The model under review builds one solid part; all positions refer to its coordinate system, in mm. A direction names the side the tool comes from. Give positions to 0.01 mm unless a question says otherwise; leave off trailing zeros. Return JSON: item names as keys, results as strings. Group by question number.
from build123d import *

# Parameters (mm, degrees)
F0_R            = 5
F1_DEPTH        = 6.5
F2_R            = 2.9
F3_DEPTH        = 10
F4_W            = 1.5
F4_H            = 25.2303039929
F5_COPIES_COUNT = 8
F6_R            = 30.1842300119
F6_R_2          = 28.1532988992
F7_DEPTH        = 4.5
F8_R            = 1.5
F9_R            = 2.5
F10_DEPTH       = 3


# Not quite as in the source:
# - a pattern or mirror of a feature is missing from the dataset's text; its kind, count and spacing are read off the source's solid


with BuildPart() as f1:
    # F0 (on Top) → F1 (new body, symmetric)
    with BuildSketch(Plane.XY):
        Circle(F0_R)
    extrude(amount=F1_DEPTH, both=True)

    # F2 (on face) → F3 (cut)
    with BuildSketch(Plane(origin=(0, 0, -6.5), x_dir=(1, 0, 0), z_dir=(0, 0, -1))):
        Circle(F2_R)
    extrude(amount=-F3_DEPTH, mode=Mode.SUBTRACT)

    # F4 (on Top) → F5 (revolve)
    with BuildSketch(Plane.XY):
        with Locations((-0.75, -17.3848480035)):
            Rectangle(F4_W, F4_H)
    f5 = revolve(axis=Axis((0, -23.260904476, 0), (0, -1, 0)))

    # F5_copies: F5 ×8 about axis
    f5_copies_axis = Axis((0, 0, 0), (0, 0, 1))
    for i in range(1, F5_COPIES_COUNT):
        add(f5.rotate(f5_copies_axis, i * 360 / F5_COPIES_COUNT))

    # F6 (on Top) → F7 (join, symmetric)
    with BuildSketch(Plane.XY):
        with Locations((0.0313063833, 0.1453618683)):
            Circle(F6_R)
        Circle(F6_R_2, mode=Mode.SUBTRACT)
    extrude(amount=F7_DEPTH, both=True)

    # F8
    f8_edges = [f1.edges().sort_by_distance(p)[0] for p in [
        (-5, 0, -6.5),
        (-28.153299, 0, -4.5),
    ]]
    fillet(f8_edges, radius=F8_R)

    # F9 (on face) → F10 (join)
    with BuildSketch(Plane.XY.offset(6.5)):
        Circle(F9_R)
    extrude(amount=F10_DEPTH)


solid = f1.part
Item 1: Tool access review of faces 4 (the face through (-0.54, -2.44, 7.98)), 5 (the face through (-2.9, -0.1, -1.6)), 6 (the face through (-16.3, -1.2, 0.9)): name each direction out of +Z, -Z, +X, -X, +Y, -Y from which nothing blocks a thin tool from reaching the whole face with its end or side.
Item 2: For P1, Ø8, axis at y = -15, z = 4.5, coming from the +X side; P2, Ø1.5, axis at x = 3, z = -3.5, coming from the -Y side; P3, Ø4.5, axis at x = -0.5, y = -0.5, coming from the -Z side; P4, Ø12, axis at x = -14.5, y = 7.5, coming from the -Z side, all flat-tipped, find the tip position at first contact; note any pin that passes through.
Item 3: Mouldability with a two-part tool opening along X and no side actions: class faces 1 (the face through (4.619, -1.915, 0.83)), 2 (the face through (-6.51, -29.32, 0.06)), 3 (the face through (2, -2, 6.5)) as +X half, -X half, draft (parallel to the pull), parting line (faces both ways), or undercut.
Item 4: For L1, parallel to Y at x = 0, z = -2; L2, parallel to X at y = 0, z = -2.25; L3, parallel to Y at x = 0, z = -0.75, list the stretches that pass through material, from the lowest coordinate up. Write a range as from..to.
Item 5: Take a section at A-A (y = -23.5). State how many separate pieces and enclosed holes the cut face has, then the cut area to 3 significant figures.
Check sheet entries:
{
 "1": {"face 4": "+Z", "face 5": "-Z", "face 6": "none"},
 "2": {"P1": "stops at x = 28.08", "P2": "stops at y = -29.96", "P3": "stops at z = -6.5", "P4": "stops at z = -1.5"},
 "3": {"face 1": "undercut", "face 2": "parting line", "face 3": "draft"},
 "4": {"L1": "y = -30.04..-28.15, -5..-2.9, 2.9..5, 28.15..30.33", "L2": "x = -30.15..-28.15, -5..-2.9, 2.9..5, 28.15..30.22", "L3": "y = -30.04..-2.9, 2.9..30.33"},
 "5": {"separate pieces": "3", "enclosed holes": "0", "area": "64.0 mm^2"}
}
